Work out the finished part from the listing and answer in its coordinate system (mm). A direction names the side the tool comes from. Coordinates: 2 decimals unless noted, no trailing zeros. Order: outer loops, then holes, each group sorted by start corner. A loop starts at its lowest first (then second) coordinate and runs counter-clockwise, first axis right, second up. Notation, with made-up numbers: M -35,25 L 8,25 A33 ccw 8,63 Z; hole C -12,-18 d7. An arc over 180 degrees is marked long. Use a Markdown table: item, result.
from build123d import *

# Parameters (mm, degrees)
SK_P01_STANDOFF_R                  = 2.5
P01_STANDOFF_DEPTH                 = 20
SK_P02_STANDOFF_R                  = 2.5
P02_STANDOFF_DEPTH                 = 20
SK_P03_STANDOFF_R                  = 2.5
P03_STANDOFF_DEPTH                 = 20
SK_P04_STANDOFF_R                  = 2.5
P04_STANDOFF_DEPTH                 = 20
P05_PERMAPROTOHAT35MMFANCUTO_START = 20
SK_P05_PERMAPROTOHAT35MMFANCUTO_W  = 65
SK_P05_PERMAPROTOHAT35MMFANCUTO_H  = 56.5
P05_PERMAPROTOHAT35MMFANCUTO_DEPTH = 2
SK_P06_STACKINGHEADER_W            = 50.8
SK_P06_STACKINGHEADER_H            = 5
P06_STACKINGHEADER_DEPTH           = 20
P07_JSTXHHEADERSVERTICAL_START     = 22
SK_P07_JSTXHHEADERSVERTICAL_W      = 8
SK_P07_JSTXHHEADERSVERTICAL_H      = 40
P07_JSTXHHEADERSVERTICAL_DEPTH     = 7


with BuildPart() as part:
    # SK_P01_Standoff → P01_Standoff (new body)
    with BuildSketch(Plane(origin=(0, 0, 0), x_dir=(1, 0, 0), z_dir=(0, 1, 0))):
        with Locations(Location((-29, 24.5, 0), (0, 0, 270))):
            Circle(SK_P01_STANDOFF_R)
    extrude(amount=P01_STANDOFF_DEPTH)



with BuildPart() as body_2:
    # SK_P02_Standoff → P02_Standoff (new body)
    with BuildSketch(Plane(origin=(0, 0, 0), x_dir=(1, 0, 0), z_dir=(0, 1, 0))):
        with Locations(Location((-29, -24.5, 0), (0, 0, 270))):
            Circle(SK_P02_STANDOFF_R)
    extrude(amount=P02_STANDOFF_DEPTH)


with BuildPart() as body_3:
    # SK_P03_Standoff → P03_Standoff (new body)
    with BuildSketch(Plane(origin=(0, 0, 0), x_dir=(1, 0, 0), z_dir=(0, 1, 0))):
        with Locations(Location((29, 24.5, 0), (0, 0, 270))):
            Circle(SK_P03_STANDOFF_R)
    extrude(amount=P03_STANDOFF_DEPTH)


with BuildPart() as body_4:
    # SK_P04_Standoff → P04_Standoff (new body)
    with BuildSketch(Plane(origin=(0, 0, 0), x_dir=(1, 0, 0), z_dir=(0, 1, 0))):
        with Locations(Location((29, -24.5, 0), (0, 0, 270))):
            Circle(SK_P04_STANDOFF_R)
    extrude(amount=P04_STANDOFF_DEPTH)


with BuildPart() as part_1:
    add(part.part)

    add(body_2.part)  # P05_PermaProtoHAT35mmfancuto merges body 2

    add(body_3.part)  # P05_PermaProtoHAT35mmfancuto merges body 3

    add(body_4.part)  # P05_PermaProtoHAT35mmfancuto merges body 4
    # SK_P05_PermaProtoHAT35mmfancuto → P05_PermaProtoHAT35mmfancuto (add)
    with BuildSketch(Plane(origin=(0, 0, 0), x_dir=(1, 0, 0), z_dir=(0, 1, 0)).offset(P05_PERMAPROTOHAT35MMFANCUTO_START)):
        Rectangle(SK_P05_PERMAPROTOHAT35MMFANCUTO_W, SK_P05_PERMAPROTOHAT35MMFANCUTO_H)
    extrude(amount=P05_PERMAPROTOHAT35MMFANCUTO_DEPTH)

    # SK_P06_Stackingheader → P06_Stackingheader (add)
    with BuildSketch(Plane(origin=(0, 0, 0), x_dir=(1, 0, 0), z_dir=(0, 1, 0))):
        with Locations((0, -24.5)):
            Rectangle(SK_P06_STACKINGHEADER_W, SK_P06_STACKINGHEADER_H)
    extrude(amount=P06_STACKINGHEADER_DEPTH)

    # SK_P07_JSTXHheadersvertical → P07_JSTXHheadersvertical (add)
    with BuildSketch(Plane(origin=(0, 0, 0), x_dir=(1, 0, 0), z_dir=(0, 1, 0)).offset(P07_JSTXHHEADERSVERTICAL_START)):
        with Locations((28.5, 2)):
            Rectangle(SK_P07_JSTXHHEADERSVERTICAL_W, SK_P07_JSTXHHEADERSVERTICAL_H)
    extrude(amount=P07_JSTXHHEADERSVERTICAL_DEPTH)


solid = part_1.part
1. Section B-B on x = -29 is taken. Determine the outline of the cut face in (y, z).
Answers below:
| item | result |
|---|---|
| outline | M 0,-27 L 20,-27 L 20,-28.25 L 22,-28.25 L 22,28.25 L 20,28.25 L 20,27 L 0,27 L 0,22 L 20,22 L 20,-22 L 0,-22 Z |
2. For faces 1 (the face through (24.5, 25, -2)), 2 (the face through (0, 10, 22)), 3 (the face through (28, 25, 18)), 4 (the face through (25.4, 10, 25)), determine the directions among +Z, -Z, +X, -X, +Y, -Y from which every point of the face is accessible in a straight line to the end or side of a thin tool.
Answers below:
| item | result |
|---|---|
| face 1 | +Z, -Z, -X, +Y |
| face 2 | -Z, +X, -X, -Y |
| face 3 | +Z, +X, -X, +Y |
| face 4 | +Z, -Z, -Y |
3. Find the intervals of material crossed by probe 1 along Z at (x, y) = (14, 11.5); probe 2 along Y at (x, z) = (-17, 16); probe 3 along Y at (x, z) = (25.5, 9), in increasing order.
Answers below:
| item | result |
|---|---|
| probe 1 | 22 to 27 |
| probe 2 | 20 to 22 |
| probe 3 | 20 to 29 |
4. For a pull along Z with two mould halves and no side action, classify faces 5 (the face through (-29, 0, -25)), 6 (the face through (28, 25, -22)), 7 (the face through (0, 21, 28.25)), 8 (the face through (31.48, 9.86, -24.83)) as +Z half, -Z half, draft (parallel to the pull), parting line (faces both ways), or undercut.
Answers below:
| item | result |
|---|---|
| face 5 | draft |
| face 6 | -Z half |
| face 7 | +Z half |
| face 8 | undercut |
5. Flat-ended cylindrical pins translate along their axes: P1, Ø5.5, axis at y = 11.5, z = 24.5, coming from the +X side; P2, Ø2, axis at x = -19.5, y = 10.5, coming from the -Z side; P3, Ø12, axis at x = -16.5, z = -12, coming from the +Y side; P4, Ø1, axis at y = 3.5, z = -20, coming from the -X side. Find the tip coordinate at first contact, or state that the pin passes through.
Answers below:
| item | result |
|---|---|
| P1 | x = 31.5 |
| P2 | z = 22 |
| P3 | y = 22 |
| P4 | through |
6. Section C-C on z = -24.5 is taken. Determine the outline of the cut face in (x, y), then the cut area to 3 significant figures.
Answers below:
| item | result |
|---|---|
| outline | M -32.5,20 L -31.5,20 L -31.5,0 L -26.5,0 L -26.5,20 L 26.5,20 L 26.5,0 L 31.5,0 L 31.5,20 L 32.5,20 L 32.5,22 L -32.5,22 Z |
| area | 330 mm² |
7. Section A-A on y = 11 is taken. Determine the outline of the cut face in (x, z).
Answers below:
| item | result |
|---|---|
| outline | C -29,-24.5 d5; C -29,24.5 d5; M -25.4,22 L 25.4,22 L 25.4,27 L -25.4,27 Z; C 29,-24.5 d5; C 29,24.5 d5 |
8. Section D-D on x = 8.5 is taken. Determine the outline of the cut face in (y, z), then the cut area to 3 significant figures.
Answers below:
| item | result |
|---|---|
| outline | M 0,22 L 20,22 L 20,-28.25 L 22,-28.25 L 22,28.25 L 20,28.25 L 20,27 L 0,27 Z |
| area | 213 mm² |
